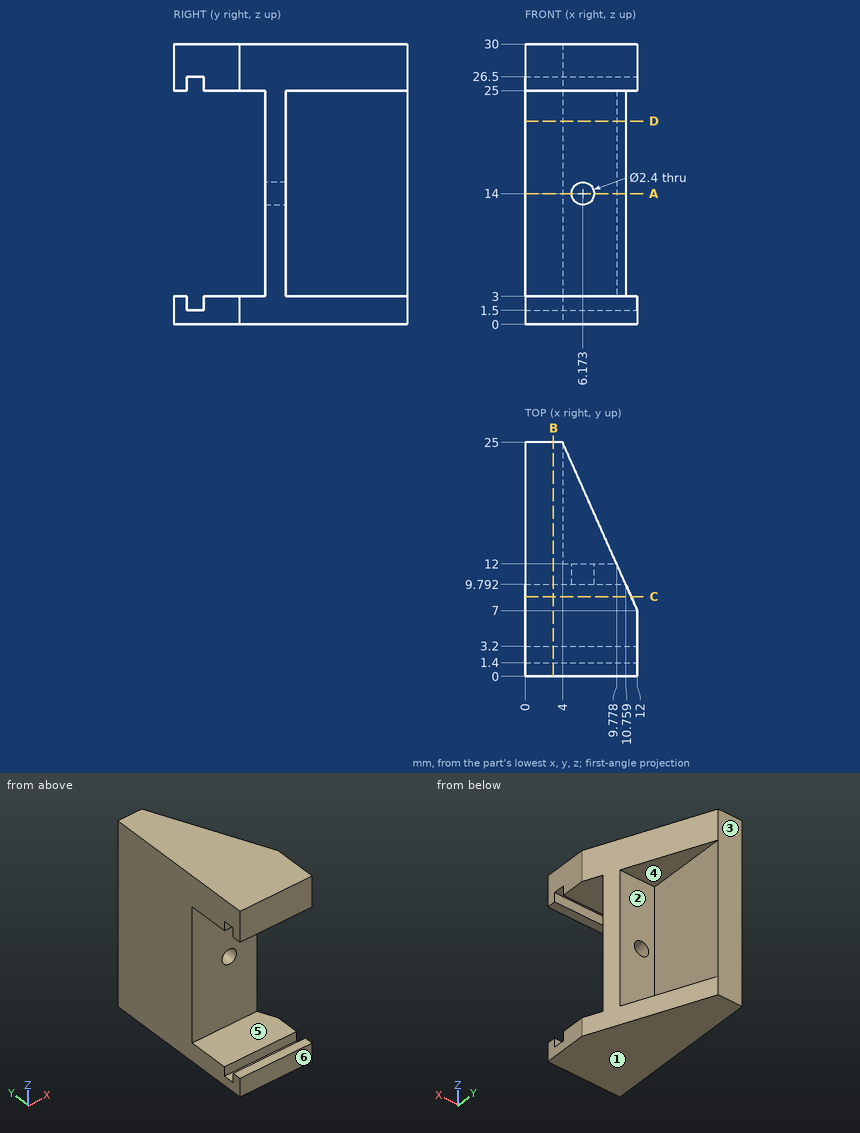
Here's the drawing with two shaded views (mm, measured from the low corner). I have some questions. A direction names the side the tool comes from. Coordinates: 2 decimals unless noted, no trailing zeros. Loops run counter-clockwise (first coordinate to the right, second up) from the corner with the lowest first, then second, coordinate; pieces in that order, holes last. Notation, with made-up numbers: (-34, 48.25) -> (-30, 48.25) arc R29 ccw to (-30, 68.25) -> close; hole circle Ø11 at (82.5, 55.5). An arc over 180 degrees is marked (long way). Put each result on its own line as item: value. Start each with the question number.
Q1. For the marked faces 4, 5 and 6, which set-ups out of +Z, -Z, +X, -X, +Y, -Y let a thin tool reach every point of the face, with its end or its side?
Q2. I want a section at D-D (z = 21.75). Write out the boundary of the cut face in (x, y).
Q3. I want a section at B-B (x = 3). Write out the boundary of the cut face in (y, z), plus the area to 3 significant figures.
Q4. Thinking about a two-plate mould opening in Z: for the marked faces 1, 2 and 3, which applies, pulls with the +Z half, pulls with the -Z half, needs draft (parallel to the pull), parting line crosses it, or undercut?
Q5. If I drill on line 1 (Z direction, x = 10.5, y = 3.5); line 2 (Z direction, x = 3.5, y = 2); line 3 (Y direction, x = 7.5, z = 5), over which ranges is the centre line in solid material (lowest first)? Write a range as [from, to].
Q6. I want a section at C-C (y = 8.5). Write out the boundary of the cut face in (x, z).
Q7. I want a section at A-A (z = 14). Write out the boundary of the cut face in (x, y).
Q8. I'm going to push flat-ended pins straight in: P1, Ø1.6, axis at x = 6.5, z = 25.5, coming from the +Y side (1 decimal); P2, Ø6, axis at x = 7, z = 14, coming from the -Y side; P3, Ø14.5, axis at y = 20, z = 15.5, coming from the +X side; P4, Ø1.5, axis at x = 6, z = 24.5, coming from the -Y side. Where does each tip first touch, or does it pass through?
Taken from the geometry:
1. face 4: +X, +Y
1. face 5: +X, -X, -Y
1. face 6: +Z, -Z, +X, -X, -Y
2. outline: (0, 9.79) -> (10.76, 9.79) -> (9.78, 12) -> (4, 12) -> (4, 25) -> (0, 25) -> close
3. outline: (0, 0) -> (25, 0) -> (25, 30) -> (0, 30) -> (0, 25) -> (1.4, 25) -> (1.4, 26.5) -> (3.2, 26.5) -> (3.2, 25) -> (9.79, 25) -> (9.79, 3) -> (3.2, 3) -> (3.2, 1.5) -> (1.4, 1.5) -> (1.4, 3) -> (0, 3) -> close
3. area: 529 mm2
4. face 1: pulls with the -Z half
4. face 2: undercut
4. face 3: needs draft
5. line 1: z = [0, 3], [25, 30]
5. line 2: z = [0, 1.5], [26.5, 30]
5. line 3: y = [9.79, 12]
6. outline: (0, 0) -> (11.33, 0) -> (11.33, 3) -> (0, 3) -> close; (0, 25) -> (11.33, 25) -> (11.33, 30) -> (0, 30) -> close
7. outline: (0, 9.79) -> (4.97, 9.79) -> (4.97, 12) -> (4, 12) -> (4, 25) -> (0, 25) -> close; (7.37, 9.79) -> (10.76, 9.79) -> (9.78, 12) -> (7.37, 12) -> close
8. P1: stops at y = 21.2
8. P2: stops at y = 9.79
8. P3: stops at x = 4
8. P4: stops at y = 0
